```python
from build123d import *

# Parameters (mm, degrees)
F2_W     = 182.88
F2_H     = 274.32
F3_DEPTH = 152.4
F4_R     = 5.159375
F5_DEPTH = 152.4
F6_W     = 60.96
F6_H     = 152.4
F7_DEPTH = 152.4
F8_R     = 0.79375


with BuildPart() as f3:
    # F2 (on Front) → F3 (new body)
    with BuildSketch(Plane.XZ):
        Rectangle(F2_W, F2_H)
    extrude(amount=-F3_DEPTH)

    # F4 (on face) → F5 (cut)
    with BuildSketch(Plane.XZ):
        with Locations((-60.96, 106.68)):
            Circle(F4_R)
        with Locations((60.96, 106.68)):
            Circle(F4_R)
        with Locations((-60.96, -106.68)):
            Circle(F4_R)
        with Locations((60.96, -106.68)):
            Circle(F4_R)
    extrude(amount=-F5_DEPTH, mode=Mode.SUBTRACT)

    # F6 (on face) → F7 (cut)
    with BuildSketch(Plane.XZ):
        Rectangle(F6_W, F6_H)
    extrude(amount=-F7_DEPTH, mode=Mode.SUBTRACT)

    # F8
    f8_edges = [f3.edges().sort_by_distance(p)[0] for p in [
        (-30.48, 76.2, 76.2),
        (30.48, 76.2, 76.2),
        (30.48, 76.2, -76.2),
        (-30.48, 76.2, -76.2),
    ]]
    fillet(f8_edges, radius=F8_R)


solid = f3.part
```
Could you check a few things on this model? Use its own coordinates, in mm. A direction names the side the tool comes from. Coordinates: 2 decimals unless noted, no trailing zeros. Write each loop counter-clockwise with the first axis right and the second up, starting at its lowest first coordinate (ties: lowest second). Pieces come first, ordered by that corner, then holes. Notation, with made-up numbers: M 43.5,-1 L 98.5,-1 A25 ccw 98.5,35 Z; hole C -4,65 d2. An arc over 180 degrees is marked long. Answer as CSV lines item,"result". Start each with the question number.
1) We'd pull the mould along X, two halves only. Please class faces 3 (the flat face through (-91.44, 75, -2)), 4 (the cylindrical face through (-62.078, 75.133, 101.643)), 5 (the flat face through (0, 75, 76.2)), 6 (the flat face through (-1, 75, -137.16)): +X half, -X half, draft (parallel to the pull), parting line (faces both ways), or undercut.
2) Please list where these lines run through material, in increasing order: line 1 (Z direction, x = 60.96, y = 60.5); line 2 (Z direction, x = -27, y = 20.5); line 3 (Z direction, x = -60, y = 114). Write a range as from..to.
3) I want a section at B-B, the plane x = 2.5. Please give me the cut outline in (y, z), and give its area (3 significant figures).
4) I want a section at C-C, the plane y = 39.5. Please give me the cut outline in (x, z).
5) For faces 1 (the flat face through (-30.48, 75, -1)), 2 (the flat face through (-1, 75, 137.16)), which set-ups out of +Z, -Z, +X, -X, +Y, -Y let a thin tool reach every point of the face, with its end or its side?
6) I want a section at D-D, the plane z = -64.5. Please give me the cut outline in (x, y), and give its area (3 significant figures).
7) I want a section at A-A, the plane z = 106.68. Please give me the cut outline in (x, y).
Data:
1,face 3,"-X half"
1,face 4,"undercut"
1,face 5,"undercut"
1,face 6,"draft"
2,line 1,"z = -137.16..-111.84, -101.52..101.52, 111.84..137.16"
2,line 2,"z = -137.16..-76.2, 76.2..137.16"
2,line 3,"z = -137.16..-111.75, -101.61..101.61, 111.75..137.16"
3,outline,"M 0,-137.16 L 152.4,-137.16 L 152.4,-76.2 L 0,-76.2 Z; M 0,76.2 L 152.4,76.2 L 152.4,137.16 L 0,137.16 Z"
3,area,"18,600 mm^2"
4,outline,"M -91.44,-137.16 L 91.44,-137.16 L 91.44,137.16 L -91.44,137.16 Z; hole C -60.96,-106.68 d10.32; hole C -60.96,106.68 d10.32; hole M -30.48,-75.41 A0.79 ccw -29.69,-76.2 L 29.69,-76.2 A0.79 ccw 30.48,-75.41 L 30.48,75.41 A0.79 ccw 29.69,76.2 L -29.69,76.2 A0.79 ccw -30.48,75.41 Z; hole C 60.96,-106.68 d10.32; hole C 60.96,106.68 d10.32"
5,face 1,"+Y, -Y"
5,face 2,"+Z, +X, -X, +Y, -Y"
6,outline,"M -91.44,0 L -30.48,0 L -30.48,152.4 L -91.44,152.4 Z; M 30.48,0 L 91.44,0 L 91.44,152.4 L 30.48,152.4 Z"
6,area,"18,600 mm^2"
7,outline,"M -91.44,0 L -66.12,0 L -66.12,152.4 L -91.44,152.4 Z; M -55.8,0 L 55.8,0 L 55.8,152.4 L -55.8,152.4 Z; M 66.12,0 L 91.44,0 L 91.44,152.4 L 66.12,152.4 Z"
